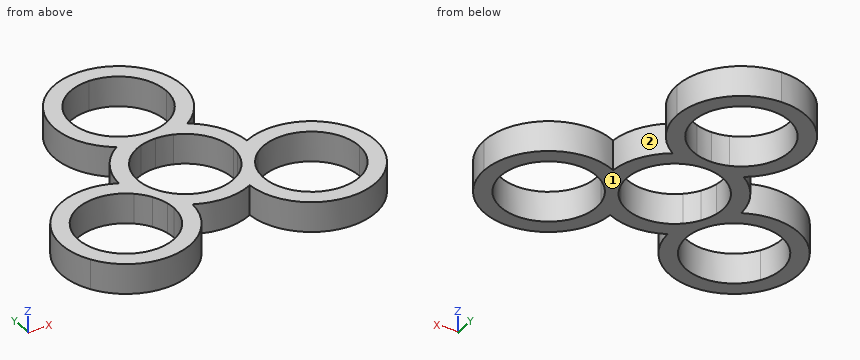
```python
from build123d import *

# Parameters (mm, degrees)
F1_DEPTH = 7


with BuildPart() as f1:
    # F0 (on Top) → F1 (new body)
    with BuildSketch(Plane.XY):
        with BuildLine():
            ThreePointArc((-3.8906200654, 10.4491901843), (-2.0298332845, 10.9636798949), (-0.1081914722, 11.1494750821))
            Line((-0.1081914722, 11.1494750821), (-0.1343903041, 13.8493479719))
            ThreePointArc((-0.1343903041, 13.8493479719), (-2.0592757302, 13.9978175054), (-3.9296961082, 14.4761005971))
            ThreePointArc((-3.9296961082, 14.4761005971), (-6.2562113602, 13.6330414588), (-8.4124625152, 12.4189562537))
            ThreePointArc((-8.4124625152, 12.4189562537), (-6.2330573108, 11.2469430781), (-3.8906200654, 10.4491901843))
        make_face()
        with BuildLine():
            Line((-0.1343903041, 13.8493479719), (-0.1081914722, 11.1494750821))
            ThreePointArc((-0.1081914722, 11.1494750821), (1.8166939539, 11.0010055485), (3.6871143319, 10.5227224568))
            ThreePointArc((3.6871143319, 10.5227224568), (6.0136295839, 11.3657815952), (8.1698807389, 12.5798668003))
            ThreePointArc((8.1698807389, 12.5798668003), (5.9904755345, 13.7518799759), (3.648038289, 14.5496328697))
            ThreePointArc((3.648038289, 14.5496328697), (1.7872515082, 14.0351431591), (-0.1343903041, 13.8493479719))
        make_face()
        with BuildLine():
            ThreePointArc((-10.9565021305, -2.0682265504), (-9.709824396, 5.4810409776), (-3.8906200654, 10.4491901843))
            ThreePointArc((-3.8906200654, 10.4491901843), (-6.2330573108, 11.2469430781), (-8.4124625152, 12.4189562537))
            ThreePointArc((-8.4124625152, 12.4189562537), (-13.0625440306, 7.3735977277), (-14.9794245947, 0.7853908656))
            ThreePointArc((-14.9794245947, 0.7853908656), (-12.8498703872, -0.474934809), (-10.9565021305, -2.0682265504))
        make_face()
        with BuildLine():
            ThreePointArc((8.1698807389, 12.5798668003), (6.0136295839, 11.3657815952), (3.6871143319, 10.5227224568))
            ThreePointArc((3.6871143319, 10.5227224568), (9.0948838585, 6.4502393444), (11.15, 0))
            ThreePointArc((11.15, 0), (11.1110756032, -0.930859248), (10.9945741812, -1.8552192791))
            ThreePointArc((10.9945741812, -1.8552192791), (12.8566670759, -0.2254855646), (14.9613628618, 1.0759281197))
            ThreePointArc((14.9613628618, 1.0759281197), (12.9169949647, 7.6256961047), (8.1698807389, 12.5798668003))
        make_face()
        with BuildLine():
            ThreePointArc((10.9945741812, -1.8552192791), (10.5097419502, -3.7239527576), (9.709824396, -5.4810409776))
            Line((9.709824396, -5.4810409776), (12.0610823215, -6.8082885686))
            ThreePointArc((12.0610823215, -6.8082885686), (13.1521034224, -5.2155236569), (14.5015189189, -3.8348336397))
            ThreePointArc((14.5015189189, -3.8348336397), (14.87485771, -1.933548062), (15, 0))
            ThreePointArc((15, 0), (14.9903376034, 0.538310818), (14.9613628618, 1.0759281197))
            ThreePointArc((14.9613628618, 1.0759281197), (12.8566670759, -0.2254855646), (10.9945741812, -1.8552192791))
        make_face()
        with BuildLine():
            Line((12.0610823215, -6.8082885686), (9.709824396, -5.4810409776))
            ThreePointArc((9.709824396, -5.4810409776), (8.6188032952, -7.0738058892), (7.2693877987, -8.4544959065))
            ThreePointArc((7.2693877987, -8.4544959065), (6.8362408033, -10.8908467862), (6.8095438558, -13.3652576659))
            ThreePointArc((6.8095438558, -13.3652576659), (8.9142396416, -12.0638439816), (10.7763325364, -10.4341102671))
            ThreePointArc((10.7763325364, -10.4341102671), (11.2611647674, -8.5653767885), (12.0610823215, -6.8082885686))
        make_face()
        with BuildLine():
            ThreePointArc((6.8095438558, -13.3652576659), (6.8362408033, -10.8908467862), (7.2693877987, -8.4544959065))
            ThreePointArc((7.2693877987, -8.4544959065), (0.1081914722, -11.1494750821), (-7.1039541159, -8.5939709052))
            ThreePointArc((-7.1039541159, -8.5939709052), (-6.6729292484, -10.6317016968), (-6.5283249412, -12.7094935078))
            ThreePointArc((-6.5283249412, -12.7094935078), (-6.5334696748, -13.1023236743), (-6.5489003466, -13.4948843734))
            ThreePointArc((-6.5489003466, -13.4948843734), (0.1455490658, -14.9992938324), (6.8095438558, -13.3652576659))
        make_face()
        with BuildLine():
            ThreePointArc((-7.1039541159, -8.5939709052), (-8.4799086657, -7.2397271373), (-9.6016329238, -5.6684341045))
            Line((-9.6016329238, -5.6684341045), (-11.9266920175, -7.0410594033))
            ThreePointArc((-11.9266920175, -7.0410594033), (-11.0928276921, -8.7822938485), (-10.5718228107, -10.6412669574))
            ThreePointArc((-10.5718228107, -10.6412669574), (-8.678454554, -12.2345586988), (-6.5489003466, -13.4948843734))
            ThreePointArc((-6.5489003466, -13.4948843734), (-6.5334696748, -13.1023236743), (-6.5283249412, -12.7094935078))
            ThreePointArc((-6.5283249412, -12.7094935078), (-6.6729292484, -10.6317016968), (-7.1039541159, -8.5939709052))
        make_face()
        with BuildLine():
            Line((-11.9266920175, -7.0410594033), (-9.6016329238, -5.6684341045))
            ThreePointArc((-9.6016329238, -5.6684341045), (-10.4354972491, -3.9271996593), (-10.9565021305, -2.0682265504))
            ThreePointArc((-10.9565021305, -2.0682265504), (-12.8498703872, -0.474934809), (-14.9794245947, 0.7853908656))
            ThreePointArc((-14.9794245947, 0.7853908656), (-14.9047151761, -1.6880359943), (-14.4243708254, -4.1155226026))
            ThreePointArc((-14.4243708254, -4.1155226026), (-13.0484162756, -5.4697663705), (-11.9266920175, -7.0410594033))
        make_face()
        with BuildLine():
            ThreePointArc((-0.3881308421, 39.9981168863), (-14.6453286848, 29.1893935987), (-8.4124625152, 12.4189562537))
            ThreePointArc((-8.4124625152, 12.4189562537), (-6.2562113602, 13.6330414588), (-3.9296961082, 14.4761005971))
            ThreePointArc((-3.9296961082, 14.4761005971), (-11.2435873248, 26.8155170078), (-0.3507732486, 36.148298136))
            Line((-0.3507732486, 36.148298136), (-0.3881308421, 39.9981168863))
        make_face()
        with BuildLine():
            ThreePointArc((3.648038289, 14.5496328697), (5.9904755345, 13.7518799759), (8.1698807389, 12.5798668003))
            ThreePointArc((8.1698807389, 12.5798668003), (13.0085868085, 17.9698450958), (14.7574182237, 24.9988230539))
            ThreePointArc((14.7574182237, 24.9988230539), (10.3124351354, 35.6567599084), (-0.3881308421, 39.9981168863))
            Line((-0.3881308421, 39.9981168863), (-0.3507732486, 36.148298136))
            ThreePointArc((-0.3507732486, 36.148298136), (7.603314128, 32.9212227824), (10.9074182237, 24.9988230539))
            ThreePointArc((10.9074182237, 24.9988230539), (8.9144623354, 18.6371374962), (3.648038289, 14.5496328697))
        make_face()
        with BuildLine():
            ThreePointArc((36.7709067176, -12.2893295462), (29.6085352544, 0.5001809573), (14.9613628618, 1.0759281197))
            ThreePointArc((14.9613628618, 1.0759281197), (14.9903376034, 0.538310818), (15, 0))
            ThreePointArc((15, 0), (14.87485771, -1.933548062), (14.5015189189, -3.8348336397))
            ThreePointArc((14.5015189189, -3.8348336397), (26.4221875114, -2.1558164842), (32.9209067176, -12.2893295462))
            ThreePointArc((32.9209067176, -12.2893295462), (32.5548540936, -15.1228748506), (31.4807311136, -17.7703705237))
            Line((31.4807311136, -17.7703705237), (34.8334507481, -19.6629272739))
            ThreePointArc((34.8334507481, -19.6629272739), (36.2784592413, -16.1012739018), (36.7709067176, -12.2893295462))
        make_face()
        with BuildLine():
            ThreePointArc((10.7763325364, -10.4341102671), (8.9142396416, -12.0638439816), (6.8095438558, -13.3652576659))
            ThreePointArc((6.8095438558, -13.3652576659), (18.4820560276, -26.9243376138), (34.8334507481, -19.6629272739))
            Line((34.8334507481, -19.6629272739), (31.4807311136, -17.7703705237))
            ThreePointArc((31.4807311136, -17.7703705237), (18.04695396, -22.7990714963), (10.7763325364, -10.4341102671))
        make_face()
        with BuildLine():
            ThreePointArc((-14.4243708254, -4.1155226026), (-14.9047151761, -1.6880359943), (-14.9794245947, 0.7853908656))
            ThreePointArc((-14.9794245947, 0.7853908656), (-32.5581883674, -2.5437612272), (-34.445319906, -20.3351896124))
            Line((-34.445319906, -20.3351896124), (-31.129957865, -18.3779276122))
            ThreePointArc((-31.129957865, -18.3779276122), (-28.7680520785, -4.2295848421), (-14.4243708254, -4.1155226026))
        make_face()
        with BuildLine():
            ThreePointArc((-34.445319906, -20.3351896124), (-17.9560920351, -27.2779234872), (-6.5489003466, -13.4948843734))
            ThreePointArc((-6.5489003466, -13.4948843734), (-8.678454554, -12.2345586988), (-10.5718228107, -10.6412669574))
            ThreePointArc((-10.5718228107, -10.6412669574), (-10.4268048031, -11.6708643043), (-10.3783249412, -12.7094935078))
            ThreePointArc((-10.3783249412, -12.7094935078), (-18.5902734696, -23.4654385406), (-31.129957865, -18.3779276122))
            Line((-31.129957865, -18.3779276122), (-34.445319906, -20.3351896124))
        make_face()
    extrude(amount=F1_DEPTH)


solid = f1.part
```
Build history of the part. All positions in model axes, mm. Face numbers are marked on the shaded views. Round coordinates to 2 decimals unless told otherwise and drop trailing zeros. Order: outer loops, then holes, each group sorted by start corner. A loop starts at its lowest first (then second) coordinate and runs counter-clockwise, first axis right, second up. Notation, with made-up numbers: (34.25, 5.5) - (53.25, 5.5) arc R12 ccw to (53.25, 22.5) - close; hole circle Ø9 at (5, -35). An arc over 180 degrees is marked (long way). Use a Markdown table: item, result.
1) Saw through at D-D on z = 3.75. Write the cut outline in (x, y).
Recorded:
| item | result |
|---|---|
| outline | (-14.98, 0.79) arc R15 ccw (long way) to (-6.55, -13.49) arc R15 ccw to (6.81, -13.37) arc R15 ccw (long way) to (14.96, 1.08) arc R15 ccw to (8.17, 12.58) arc R15 ccw (long way) to (-8.41, 12.42) arc R15 ccw to start; hole circle Ø22.3 at (-21.53, -12.71); hole circle Ø22.3 at (-0.24, 25); hole circle Ø22.3 at (0, 0); hole circle Ø22.3 at (21.77, -12.29) |
2) Pull direction Y, two halves, no side cores. Call the marked faces 1 and 2: pulls with the +Y half, pulls with the -Y half, needs draft (parallel to the pull), parting line crosses it, or undercut.
Recorded:
| item | result |
|---|---|
| face 1 | needs draft |
| face 2 | undercut |
3) Wall check: L1, parallel to Y at x = 0, z = 1; L2, parallel to Y at x = -10, z = 5; L3, parallel to X at y = 1, z = 6. Give the ranges that are in metal, low to high.
Recorded:
| item | result |
|---|---|
| L1 | y = -15 to -11.15, 11.15 to 13.85, 36.15 to 40 |
| L2 | y = -22.31 to -4.93, 4.93 to 11.18, 13.61 to 19.6, 30.39 to 36.39 |
| L3 | x = -27.62 to -15.44, -14.97 to -11.11, 11.11 to 28.73 |
4) Saw through at C-C on y = -3. Write the cut outline in (x, z).
Recorded:
| item | result |
|---|---|
| outline | (-32.96, 0) - (-27.01, 0) - (-27.01, 7) - (-32.96, 7) - close; (-16.05, 0) - (-10.74, 0) - (-10.74, 7) - (-16.05, 7) - close; (10.74, 0) - (15.6, 0) - (15.6, 7) - (10.74, 7) - close; (27.94, 0) - (33.55, 0) - (33.55, 7) - (27.94, 7) - close |
5) Saw through at A-A on x = -16.5. Write the cut outline in (y, z).
Recorded:
| item | result |
|---|---|
| outline | (-26.84, 0) - (-22.66, 0) - (-22.66, 7) - (-26.84, 7) - close; (-2.76, 0) - (1.42, 0) - (1.42, 7) - (-2.76, 7) - close |
6) Saw through at B-B on y = 26.5. Write the cut outline in (x, z), and give its area (3 significant figures).
Recorded:
| item | result |
|---|---|
| outline | (-15.17, 0) - (-11.29, 0) - (-11.29, 7) - (-15.17, 7) - close; (10.81, 0) - (14.68, 0) - (14.68, 7) - (10.81, 7) - close |
| area | 54.3 mm² |
7) Flat gauge pins, fed straight in: pin 1 Ø2 at (x, z) = (0.5, 2.5) entering from -Y; pin 2 Ø1 at (x, z) = (11, 4) entering from +Y. Where does each tip first touch, or does it go through?
Recorded:
| item | result |
|---|---|
| pin 1 | stops at y = -15 |
| pin 2 | stops at y = 35.47 |
